Verification items for the finished model (mm, model axes). A direction names the side the tool comes from. Give positions to 0.01 mm unless a question says otherwise; leave off trailing zeros. Order: outer loops, then holes, each group sorted by start corner. A loop starts at its lowest first (then second) coordinate and runs counter-clockwise, first axis right, second up. Notation, with made-up numbers: (32, 29) - (39, 29) arc R15 ccw to (39, 37) - close; hole circle Ø6 at (16, -21). An arc over 180 degrees is marked (long way). Answer as a JSON object with one key per item and string values.
```python
from build123d import *

# Parameters (mm, degrees)
SKETCH1_R           = 3.5
BOSS_EXTRUDE1_DEPTH = 3
SKETCH2_R           = 2
BOSS_EXTRUDE2_DEPTH = 10
CHAMFER1_SIZE       = 0.3
CUT_EXTRUDE1_DEPTH  = 2


with BuildPart() as part:
    # Sketch1 → Boss-Extrude1 (new body)
    with BuildSketch(Plane.XY):
        Circle(SKETCH1_R)
    extrude(amount=BOSS_EXTRUDE1_DEPTH)

    # Sketch2 → Boss-Extrude2 (add)
    with BuildSketch(Plane(origin=(0, 0, 0), x_dir=(-1, 0, 0), z_dir=(0, 0, -1))):
        Circle(SKETCH2_R)
    extrude(amount=BOSS_EXTRUDE2_DEPTH)

    # Chamfer1
    chamfer1_edges = [part.edges().sort_by_distance(p)[0] for p in [
        (2, 0, -10),
    ]]
    chamfer(chamfer1_edges, length=CHAMFER1_SIZE)

    # Sketch3 → Cut-Extrude1 (cut)
    with BuildSketch(Plane.XY.offset(3)):
        Polygon((0, 1.732050808), (-1.5, 0.866025404), (-1.5, -0.866025404), (0, -1.732050808), (1.5, -0.866025404), (1.5, 0.866025404), align=None)
    extrude(amount=-CUT_EXTRUDE1_DEPTH, mode=Mode.SUBTRACT)


solid = part.part
```
(1) Section check D-D (y = 3). Record the cut outline in (x, z).
Computed values:
{"outline": "(-1.8, 0) - (1.8, 0) - (1.8, 3) - (-1.8, 3) - close"}
(2) Gauge pin test, flat ends, axial feed: pin 1 Ø1 at (x, z) = (-1, 1.5) entering from -Y; pin 2 Ø0.5 at (y, z) = (0.5, 2.5) entering from +X; pin 3 Ø2 at (x, z) = (0, -3) entering from -Y. Record the tip position at first contact, or that the pin passes through.
Computed values:
{"pin 1": "stops at y = -3.46", "pin 2": "stops at x = 3.49", "pin 3": "stops at y = -2"}
(3) Section check A-A (y = 0). Record the cut outline in (x, z).
Computed values:
{"outline": "(-3.5, 0) - (-2, 0) - (-2, -9.7) - (-1.7, -10) - (1.7, -10) - (2, -9.7) - (2, 0) - (3.5, 0) - (3.5, 3) - (1.5, 3) - (1.5, 1) - (-1.5, 1) - (-1.5, 3) - (-3.5, 3) - close"}
(4) Material ranges on line 1 along X through (y, z) = (-1, -0.25); line 2 along Z through (x, y) = (-1.5, 1.75); line 3 along Y through (x, z) = (1.25, -7.5), recorded low to high. Write a range as [from, to].
Computed values:
{"line 1": "x = [-1.73, 1.73]", "line 2": "z = [0, 3]", "line 3": "y = [-1.56, 1.56]"}
(5) Release check for a two-part mould opening along X. For faces 1 (the cylindrical face through (0, -2, -5)), 2 (the flat face through (0.76, 1.293, 2.014)), 3 (the flat face through (2, -2, 0)) record: pulls with the +X half, pulls with the -X half, needs draft (parallel to the pull), parting line crosses it, or undercut.
Computed values:
{"face 1": "parting line crosses it", "face 2": "undercut", "face 3": "needs draft"}
(6) Section check C-C (x = -2.25). Record the cut outline in (y, z), then the cut area to 3 significant figures.
Computed values:
{"outline": "(-2.68, 0) - (2.68, 0) - (2.68, 3) - (-2.68, 3) - close", "area": "16.1 mm²"}
(7) Access from +Z, -Z, +X, -X, +Y, -Y to the whole of each face (thin tool, end or side, straight path). Record for faces 4 (the flat face through (-1.5, 0, 2)), 5 (the cylindrical face through (3.233, -1.341, 1.479)).
Computed values:
{"face 4": "+Z", "face 5": "+Z, -Z"}
(8) Section check B-B (z = -7.5). Record the cut outline in (x, y), then the cut area to 3 significant figures.
Computed values:
{"outline": "circle Ø4 at (0, 0)", "area": "12.6 mm²"}
